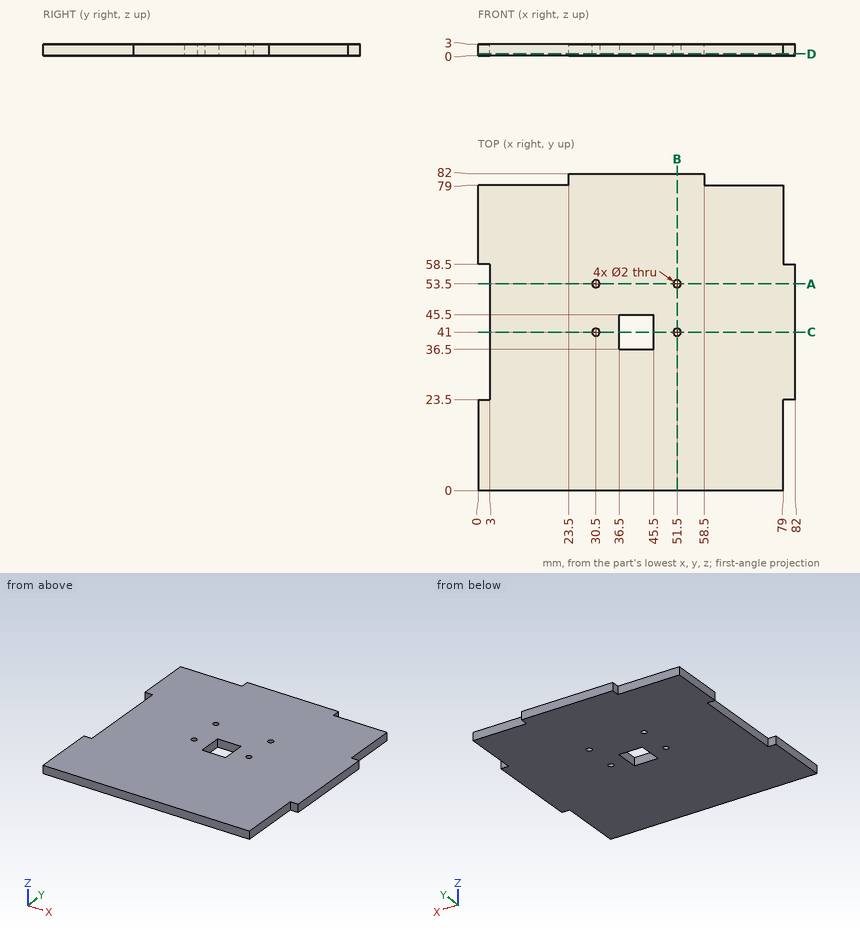
Part print with two shaded views. Sizes in mm from the minimum x, y, z corner. Give positions to 0.01 mm unless a question says otherwise; leave off trailing zeros. Order: outer loops, then holes, each group sorted by start corner. A loop starts at its lowest first (then second) coordinate and runs counter-clockwise, first axis right, second up. Notation, with made-up numbers: M 54,27.5 L 90,27.5 A35 ccw 90,63.5 Z; hole C 33,-21.75 d5. An arc over 180 degrees is marked long. Write item = value, one per line.
Q1. Cut at C-C, the plane y = 41. List the corners of the cut face in (x, z).
Derived:
outline = M 3,0 L 29.5,0 L 29.5,3 L 3,3 Z; M 31.5,0 L 36.5,0 L 36.5,3 L 31.5,3 Z; M 45.5,0 L 50.5,0 L 50.5,3 L 45.5,3 Z; M 52.5,0 L 82,0 L 82,3 L 52.5,3 Z
Q2. Cut at B-B, the plane x = 51.5. List the corners of the cut face in (y, z).
Derived:
outline = M 0,0 L 40,0 L 40,3 L 0,3 Z; M 42,0 L 52.5,0 L 52.5,3 L 42,3 Z; M 54.5,0 L 82,0 L 82,3 L 54.5,3 Z
Q3. Drill centre lines: line 1 (Y direction, x = 30.5, z = 1.45); line 2 (X direction, y = 18, z = 2.2). Where is each one in solid material? Low to high. Write a range as [from, to].
Derived:
line_1 = [0, 40], [42, 52.5], [54.5, 82]
line_2 = [0, 79]
Q4. Flat gauge pins, fed straight in: pin 1 (0.9 mm diameter, centred on y = 6.5, z = 1.5, fed in from +X); pin 2 (0.9 mm diameter, centred on y = 34, z = 2, fed in from -X); pin 3 (0.9 mm diameter, centred on x = 70, z = 1.5, fed in from +Y). Where does each tip first touch, or does it go through?
Derived:
pin_1 = 79
pin_2 = 3
pin_3 = 79
Q5. Cut at D-D, the plane z = 0.45. List the corners of the cut face in (x, y).
Derived:
outline = M 0,0 L 79,0 L 79,23.5 L 82,23.5 L 82,58.5 L 79,58.5 L 79,79 L 58.5,79 L 58.5,82 L 23.5,82 L 23.5,79 L 0,79 L 0,58.5 L 3,58.5 L 3,23.5 L 0,23.5 Z; hole C 30.5,41 d2; hole C 30.5,53.5 d2; hole M 36.5,36.5 L 45.5,36.5 L 45.5,45.5 L 36.5,45.5 Z; hole C 51.5,41 d2; hole C 51.5,53.5 d2
Q6. Cut at A-A, the plane y = 53.5. List the corners of the cut face in (x, z), then the cut area to 3 significant figures.
Derived:
outline = M 3,0 L 29.5,0 L 29.5,3 L 3,3 Z; M 31.5,0 L 50.5,0 L 50.5,3 L 31.5,3 Z; M 52.5,0 L 82,0 L 82,3 L 52.5,3 Z
area = 225 mm2
